from build123d import *

# Parameters (mm, degrees)
BOSS_EXTRUDE1_DEPTH     = 93
SKETCH2_W               = 42.5
SKETCH2_H               = 42.6
CUT_EXTRUDE1_DEPTH      = 3.5
SKETCH3_R               = 11.5
CUT_EXTRUDE2_DEPTH      = 12.5
SKETCH4_R               = 1.75
CUT_EXTRUDE3_DEPTH      = 12.5
CUT_EXTRUDE4_START      = -11.5
SKETCH4_3_R             = 3
SKETCH4_3_R_2           = 1.75
CUT_EXTRUDE4_DEPTH      = 3
SKETCH5_R               = 3.25
CUT_EXTRUDE5_DEPTH      = 51
CUT_EXTRUDE5_DEPTH_BACK = 14
SKETCH5_3_R             = 6.25
SKETCH5_3_R_2           = 3.25
CUT_EXTRUDE6_DEPTH      = 51
CUT_EXTRUDE6_DEPTH_BACK = 7
CUT_EXTRUDE7_DEPTH      = 14


with BuildPart() as part:
    # Sketch1 → Boss-Extrude1 (new body)
    with BuildSketch(Plane(origin=(0, 0, 0), x_dir=(0, 0, -1), z_dir=(1, 0, 0))):
        Polygon((0, 0), (-50, 0), (-50, -15), (13, -15), (13, 86.965010888), (0, 86.965010888), align=None)
    extrude(amount=-BOSS_EXTRUDE1_DEPTH)

    # Sketch2 → Cut-Extrude1 (cut)
    with BuildSketch(Plane(origin=(0, 0, 0), x_dir=(1, 0, 0), z_dir=(0, 1, 0))):
        with Locations((-46.5, -25.3)):
            Rectangle(SKETCH2_W, SKETCH2_H)
    extrude(amount=-CUT_EXTRUDE1_DEPTH, mode=Mode.SUBTRACT)

    # Sketch3 → Cut-Extrude2 (cut, through all)
    with BuildSketch(Plane(origin=(0, -3.5, 0), x_dir=(1, 0, 0), z_dir=(0, 1, 0))):
        with Locations((-46.5, -25.3)):
            Circle(SKETCH3_R)
    extrude(amount=-CUT_EXTRUDE2_DEPTH, mode=Mode.SUBTRACT)

    # Sketch4 → Cut-Extrude3 (cut, through all)
    with BuildSketch(Plane(origin=(0, -3.5, 0), x_dir=(1, 0, 0), z_dir=(0, 1, 0))):
        with Locations((-62, -9.8)):
            Circle(SKETCH4_R)
        with Locations((-31, -9.8)):
            Circle(SKETCH4_R)
        with Locations((-31, -40.8)):
            Circle(SKETCH4_R)
        with Locations((-62, -40.8)):
            Circle(SKETCH4_R)
    extrude(amount=-CUT_EXTRUDE3_DEPTH, mode=Mode.SUBTRACT)

    # Sketch4_3 → Cut-Extrude4 (cut)
    with BuildSketch(Plane(origin=(0, -3.5, 0), x_dir=(1, 0, 0), z_dir=(0, 1, 0)).offset(CUT_EXTRUDE4_START)):
        with Locations((-62, -9.8)):
            Circle(SKETCH4_3_R)
        with Locations((-62, -9.8)):
            Circle(SKETCH4_3_R_2, mode=Mode.SUBTRACT)
        with Locations((-31, -9.8)):
            Circle(SKETCH4_3_R)
        with Locations((-31, -9.8)):
            Circle(SKETCH4_3_R_2, mode=Mode.SUBTRACT)
        with Locations((-31, -40.8)):
            Circle(SKETCH4_3_R)
        with Locations((-31, -40.8)):
            Circle(SKETCH4_3_R_2, mode=Mode.SUBTRACT)
        with Locations((-62, -40.8)):
            Circle(SKETCH4_3_R)
        with Locations((-62, -40.8)):
            Circle(SKETCH4_3_R_2, mode=Mode.SUBTRACT)
    extrude(amount=CUT_EXTRUDE4_DEPTH, mode=Mode.SUBTRACT)

    # Sketch5 → Cut-Extrude5 (cut, two sides)
    with BuildSketch(Plane.XY) as cut_extrude5_sk:
        with Locations((-84.6, 68.5)):
            Circle(SKETCH5_R)
        with Locations((-8.4, 68.5)):
            Circle(SKETCH5_R)
        with Locations((-8.4, 8.5)):
            Circle(SKETCH5_R)
        with Locations((-84.6, 8.5)):
            Circle(SKETCH5_R)
    extrude(amount=CUT_EXTRUDE5_DEPTH, mode=Mode.SUBTRACT)
    extrude(cut_extrude5_sk.sketch, amount=-CUT_EXTRUDE5_DEPTH_BACK, mode=Mode.SUBTRACT)

    # Sketch5_3 → Cut-Extrude6 (cut, two sides)
    with BuildSketch(Plane.XY) as cut_extrude6_sk:
        with Locations((-84.6, 68.5)):
            Circle(SKETCH5_3_R)
        with Locations((-84.6, 68.5)):
            Circle(SKETCH5_3_R_2, mode=Mode.SUBTRACT)
        with Locations((-84.6, 8.5)):
            Circle(SKETCH5_3_R)
        with Locations((-84.6, 8.5)):
            Circle(SKETCH5_3_R_2, mode=Mode.SUBTRACT)
        with Locations((-8.4, 8.5)):
            Circle(SKETCH5_3_R)
        with Locations((-8.4, 8.5)):
            Circle(SKETCH5_3_R_2, mode=Mode.SUBTRACT)
        with Locations((-8.4, 68.5)):
            Circle(SKETCH5_3_R)
        with Locations((-8.4, 68.5)):
            Circle(SKETCH5_3_R_2, mode=Mode.SUBTRACT)
    extrude(amount=CUT_EXTRUDE6_DEPTH, mode=Mode.SUBTRACT)
    extrude(cut_extrude6_sk.sketch, amount=-CUT_EXTRUDE6_DEPTH_BACK, mode=Mode.SUBTRACT)

    # Sketch7 → Cut-Extrude7 (cut, through all)
    with BuildSketch(Plane.XY):
        with BuildLine():
            Line((-93, 86.965010888), (-93, 68.5))
            ThreePointArc((-93, 68.5), (-84.6, 76.9), (-76.2, 68.5))
            Line((-76.2, 68.5), (-76.2, 25.508589177))
            ThreePointArc((-76.2, 25.508589177), (-71.526556974, 22.245442635), (-68.033447852, 17.741290803))
            Line((-68.033447852, 17.741290803), (-24.966552148, 17.741290803))
            ThreePointArc((-24.966552148, 17.741290803), (-21.473443026, 22.245442635), (-16.8, 25.508589177))
            Line((-16.8, 25.508589177), (-16.8, 68.5))
            ThreePointArc((-16.8, 68.5), (-8.4, 76.9), (0, 68.5))
            Line((0, 68.5), (0, 86.965010888))
            Line((0, 86.965010888), (-93, 86.965010888))
        make_face()
    extrude(amount=-CUT_EXTRUDE7_DEPTH, mode=Mode.SUBTRACT)


solid = part.part
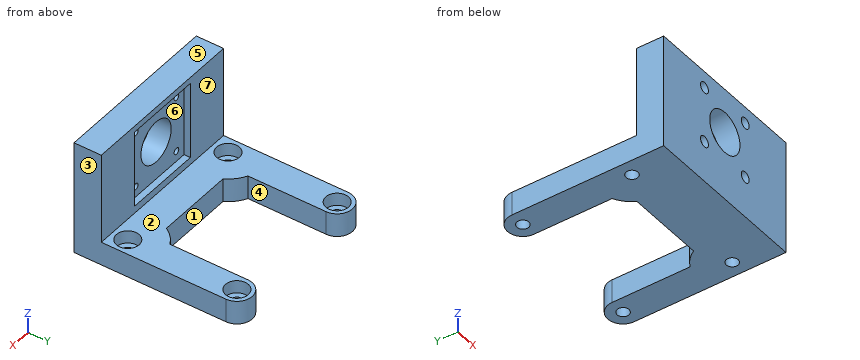
Part model, mm, in its own coordinate system. Face numbers are marked on the shaded views. A direction names the side the tool comes from. Coordinates: 2 decimals unless noted, no trailing zeros. Loops run counter-clockwise (first coordinate to the right, second up) from the corner with the lowest first, then second, coordinate; pieces in that order, holes last. Notation, with made-up numbers: (22.5, -17.5) - (32.5, -17.5) arc R17 ccw to (32.5, -6.5) - close; hole circle Ø8 at (-16, 17.25). An arc over 180 degrees is marked (long way). Write each question's results on one line, items separated by ' | '. Start each with the question number.
Q1. Slice it at C-C on z = 9.8. Give the cut face in (x, y).
Q2. Probe line 1 along Z through (x, y) = (-31, -7.5); line 2 along X through (y, z) = (-6.75, 40.8); line 3 along Z through (x, y) = (-62, -14.05). List the from-to ranges inside material, lowest first.
Q3. Two-plate mould, pull along X, no slides. Class the marked faces 1, 2 and 3: +X half, -X half, draft (parallel to the pull), parting line (faces both ways), or undercut.
Q4. Slice it at D-D on y = 8.5. Give the cut face in (x, z), and give its area (3 significant figures).
Q5. Slice it at B-B on x = -84.6. Give the cut face in (y, z).
Q6. Slice it at A-A on y = 48. Give the cut face in (x, z).
Q7. Drop flat-ended pins along their axis: pin 1 Ø25 at (x, z) = (-37.5, 36) entering from +Y; pin 2 Ø12 at (x, z) = (-57.5, 26) entering from +Y; pin 3 Ø2 at (x, y) = (-76.5, 53) entering from +Z; pin 4 Ø8 at (x, z) = (-62, 40.8) entering from -Y. Give the stop position or say it passes through.
Q8. Which spindle directions (+Z, -Z, +X, -X, +Y, -Y) get a long thin tool onto all of the face, cutting with end or side? Do the marked faces 4, 5, 6 and 7. Say none if no direction does.
Answer:
1) outline: (-93, -15) - (-65, -15) - (-65, -12) - (-63.75, -12) - (-63.75, -3.5) - (-67.75, -3.5) - (-67.75, 0) - (-93, 0) - close; (-60.25, -12) - (-59, -12) - (-59, -15) - (-34, -15) - (-34, -12) - (-32.75, -12) - (-32.75, -3.5) - (-60.25, -3.5) - close; (-29.25, -12) - (-28, -12) - (-28, -15) - (0, -15) - (0, 0) - (-25.25, 0) - (-25.25, -3.5) - (-29.25, -3.5) - close
2) line 1: z = -13 to 8.05, 11.55 to 39.05, 42.55 to 50 | line 2: x = -93 to -63.75, -60.25 to -32.75, -29.25 to 0 | line 3: z = -13 to 6.8, 12.8 to 37.8, 43.8 to 50
3) face 1: undercut | face 2: draft | face 3: +X half
4) outline: (-93, -13) - (-87.85, -13) - (-87.85, -7) - (-90.85, -7) - (-90.85, 0) - (-93, 0) - close; (-81.35, -13) - (-11.65, -13) - (-11.65, -7) - (-14.65, -7) - (-14.65, 0) - (-78.35, 0) - (-78.35, -7) - (-81.35, -7) - close; (-5.15, -13) - (0, -13) - (0, 0) - (-2.15, 0) - (-2.15, -7) - (-5.15, -7) - close | area: 956 mm2
5) outline: (-15, -13) - (5.25, -13) - (5.25, -7) - (2.25, -7) - (2.25, 0) - (0, 0) - (0, 50) - (-15, 50) - close; (11.75, -13) - (65.25, -13) - (65.25, -7) - (62.25, -7) - (62.25, 0) - (14.75, 0) - (14.75, -7) - (11.75, -7) - close; (71.75, -13) - (76.9, -13) - (76.9, 0) - (74.75, 0) - (74.75, -7) - (71.75, -7) - close
6) outline: (-93, -13) - (-76.2, -13) - (-76.2, 0) - (-93, 0) - close; (-16.8, -13) - (0, -13) - (0, 0) - (-16.8, 0) - close
7) pin 1: stops at y = 0 | pin 2: stops at y = -3.5 | pin 3: stops at z = 0 | pin 4: stops at y = -15
8) face 4: +Z, -Z, +Y | face 5: +Z, +X, -X, +Y, -Y | face 6: +Y | face 7: +Z, +X, -X, +Y
